from build123d import *

# Parameters (mm, degrees)
BOSS_EXTRUDE2_DEPTH      = 6.35
FILLET1_R                = 0.254
CIRPATTERN3_COUNT        = 3
FILLET1_OF_CIRPATTERN3_R = 0.254
CUT_EXTRUDE1_DEPTH       = 22.220069761
CUT_EXTRUDE1_DEPTH_BACK  = 22.220069761
SKETCH6_R                = 0.79375


with BuildPart() as part:
    # Sketch3 → Revolve1 (revolve)
    with BuildSketch(Plane.XY, mode=Mode.PRIVATE) as revolve1_sk:
        Polygon((0, 9.9568), (0, 2.4511), (15.875, 2.4511), (15.875, 4.0386), (3.175, 5.98805), (3.175, 9.9568), align=None)
    revolve(revolve1_sk.sketch.rotate(Axis((0, 0, 0), (1, 0, 0)), 90), axis=Axis((0, 0, 0), (1, 0, 0)))

    # Sketch5 → Boss-Extrude2 (add)
    with BuildSketch(Plane.ZY.offset(-15.875)):
        with BuildLine():
            ThreePointArc((-0.381, 2.421307541), (0, 2.4511), (0.381, 2.421307541))
            ThreePointArc((0.381, 2.421307541), (0, 2.3241), (-0.381, 2.421307541))
        make_face()
    boss_extrude2 = extrude(amount=BOSS_EXTRUDE2_DEPTH)

    # Fillet1
    # the kernel refuses this fillet: 0.254 mm, written as the material it takes off along each edge
    with BuildSketch(Plane(origin=(9.525, 3.119358803, 0), x_dir=(0, -0.2692049658318269, 0.9630829073197619), z_dir=(0, 0.9630829073197619, 0.2692049658318269))) as fillet1_piece_1_section:
        with BuildLine():
            CenterArc((0.795258803 - FILLET1_R, FILLET1_R), FILLET1_R, 270, 90)
            Line((0.795258803 - FILLET1_R, 0), (0.795258803, 0))
            Line((0.795258803, 0), (0.795258803, FILLET1_R))
        make_face()
    fillet1_piece_1 = revolve(axis=Axis((9.525, 3.119358803, 0), (1, 0, 0)), revolution_arc=148.766073655, mode=Mode.PRIVATE)
    fillet1_piece_1 = fillet1_piece_1 & Plane(origin=(9.597702858, 0, 0), x_dir=(0, 0, 1), z_dir=(1, 0, 0)) * Cylinder(2.4511, 4, mode=Mode.PRIVATE)
    add(fillet1_piece_1, mode=Mode.SUBTRACT)

    # CirPattern3: Boss-Extrude2 ×3 about axis
    cirpattern3_axis = Axis((0, 0, 0), (1, 0, 0))
    for i in range(1, CIRPATTERN3_COUNT):
        add(boss_extrude2.rotate(cirpattern3_axis, i * 360 / CIRPATTERN3_COUNT))

    # Fillet1 of CirPattern3
    # the kernel refuses this fillet: 0.254 mm, written as the material it takes off along each edge
    with BuildSketch(Plane(origin=(9.525, -1.559679402, 2.701443967), x_dir=(0, -0.699451780773575, -0.7146797928951643), z_dir=(0, -0.7146797928951643, 0.699451780773575))) as fillet1_of_cirpattern3_piece_1_section:
        with BuildLine():
            CenterArc((0.795258803 - FILLET1_OF_CIRPATTERN3_R, FILLET1_OF_CIRPATTERN3_R), FILLET1_OF_CIRPATTERN3_R, 270, 90)
            Line((0.795258803 - FILLET1_OF_CIRPATTERN3_R, 0), (0.795258803, 0))
            Line((0.795258803, 0), (0.795258803, FILLET1_OF_CIRPATTERN3_R))
        make_face()
    fillet1_of_cirpattern3_piece_1 = revolve(axis=Axis((9.525, -1.559679402, 2.701443967), (1, 0, 0)), revolution_arc=148.766073655, mode=Mode.PRIVATE)
    fillet1_of_cirpattern3_piece_1 = fillet1_of_cirpattern3_piece_1 & Plane(origin=(9.597702858, 0, 0), x_dir=(0, 0, 1), z_dir=(1, 0, 0)) * Cylinder(2.4511, 4, mode=Mode.PRIVATE)
    add(fillet1_of_cirpattern3_piece_1, mode=Mode.SUBTRACT)
    with BuildSketch(Plane(origin=(9.525, -1.559679402, -2.701443967), x_dir=(0, 0.968656746605401, -0.24840311442459811), z_dir=(0, -0.24840311442459811, -0.968656746605401))) as fillet1_of_cirpattern3_piece_2_section:
        with BuildLine():
            CenterArc((0.795258803 - FILLET1_OF_CIRPATTERN3_R, FILLET1_OF_CIRPATTERN3_R), FILLET1_OF_CIRPATTERN3_R, 270, 90)
            Line((0.795258803 - FILLET1_OF_CIRPATTERN3_R, 0), (0.795258803, 0))
            Line((0.795258803, 0), (0.795258803, FILLET1_OF_CIRPATTERN3_R))
        make_face()
    fillet1_of_cirpattern3_piece_2 = revolve(axis=Axis((9.525, -1.559679402, -2.701443967), (1, 0, 0)), revolution_arc=148.766073655, mode=Mode.PRIVATE)
    fillet1_of_cirpattern3_piece_2 = fillet1_of_cirpattern3_piece_2 & Plane(origin=(9.597702858, 0, 0), x_dir=(0, 0, 1), z_dir=(1, 0, 0)) * Cylinder(2.4511, 4, mode=Mode.PRIVATE)
    add(fillet1_of_cirpattern3_piece_2, mode=Mode.SUBTRACT)

    # Sketch6 → Cut-Extrude1 (cut, two sides: drawn at the far end of the back side and taken through both)
    with BuildSketch(Plane.XY.offset(-CUT_EXTRUDE1_DEPTH_BACK)):
        with Locations((7.9375, 0)):
            Circle(SKETCH6_R)
    extrude(amount=CUT_EXTRUDE1_DEPTH + CUT_EXTRUDE1_DEPTH_BACK, mode=Mode.SUBTRACT)


solid = part.part
Can you work these out from the model? Positions are in its coordinate system, mm. A direction names the side the tool comes from. Coordinates: 2 decimals unless noted, no trailing zeros. Write each loop counter-clockwise with the first axis right and the second up, starting at its lowest first coordinate (ties: lowest second). Pieces come first, ordered by that corner, then holes. Notation, with made-up numbers: (17.5, 83) -> (56.5, 83) arc R27 cw to (56.5, 102) -> close; hole circle Ø5 at (48, -17.5). An arc over 180 degrees is marked (long way). Write each question's results on one line, items separated by ' | '. Start each with the question number.
Q1. We'd pull the mould along X, two halves only. Please class faces 1 (the face through (7.145, 0.035, 3.827)), 2 (the face through (7.145, 0.035, -3.87)), 3 (the face through (0, 2, 2)), 4 (the face through (10.85, -1.44, 4.59)): +X half, -X half, draft (parallel to the pull), parting line (faces both ways), or undercut.
Q2. On a 3-axis mill with a long thin cutter (end or side, diameter ignored), from which of +Z, -Z, +X, -X, +Y, -Y can I reach the whole of each face in a straight line? I mean faces 5 (the face through (3.175, -0.1, -6.5)), 6 (the face through (1.565, -2.991, 9.497)). Say none if no direction works.
Q3. I'm going to push flat-ended pins straight in: pin 1 (4 mm diameter, centred on y = 6, z = -5, fed in from -X); pin 2 (2.5 mm diameter, centred on x = 7.94, y = 0, fed in from -Z); pin 3 (5 mm diameter, centred on x = 4.5, y = -7, fed in from +Z); pin 4 (2.5 mm diameter, centred on x = 7.94, y = 0, fed in from +Z). Where does each tip first touch, or does it pass through?
Q4. Imagine slicing it at B-B (y = 0). Write out the boundary of the cut face in (x, z) (3 decimals).
Q5. Imagine slicing it at D-D (y = -7.5). Write out the boundary of the cut face in (x, z) (3 decimals).
Q6. Imagine slicing it at A-A (z = 0). Write out the boundary of the cut face in (x, y) (3 decimals).
Q7. Imagine slicing it at C-C (x = 5.5). Write out the boundary of the cut face in (y, z), then the cut area to 3 significant figures.
Q8. If I drill on probe 1 along X at (y, z) = (0, -3) (3 decimals); probe 2 along X at (y, z) = (3.5, 7) (3 decimals); probe 3 along Y at (x, z) = (9, 0), over which ranges is the centre line in solid material (lowest first)?
Taken from the geometry:
1) face 1: undercut | face 2: undercut | face 3: -X half | face 4: +X half
2) face 5: +X | face 6: +X, -X
3) pin 1: stops at x = 0 | pin 2: stops at z = -5.45 | pin 3: stops at z = 8.68 | pin 4: stops at z = 5.45
4) outline: (0, -9.957) -> (3.175, -9.957) -> (3.175, -5.988) -> (7.144, -5.379) -> (7.144, -2.451) -> (0, -2.451) -> close; (0, 2.451) -> (7.144, 2.451) -> (7.144, 5.379) -> (3.175, 5.988) -> (3.175, 9.957) -> (0, 9.957) -> close; (8.731, -5.135) -> (15.875, -4.039) -> (15.875, -2.451) -> (8.731, -2.451) -> close; (8.731, 2.451) -> (15.875, 2.451) -> (15.875, 4.039) -> (8.731, 5.135) -> close
5) outline: (0, -6.549) -> (3.175, -6.549) -> (3.175, 6.549) -> (0, 6.549) -> close
6) outline: (0, -9.957) -> (3.175, -9.957) -> (3.175, -5.988) -> (15.875, -4.039) -> (15.875, -2.451) -> (0, -2.451) -> close; (0, 2.451) -> (9.559, 2.451) arc R0.254 ccw to (9.779, 2.324) -> (15.875, 2.324) -> (15.875, 4.039) -> (3.175, 5.988) -> (3.175, 9.957) -> (0, 9.957) -> close
7) outline: circle Ø11.26 at (0, 0); hole circle Ø4.9 at (0, 0) | area: 80.7 mm^2
8) probe 1: x = 0 to 7.144, 8.731 to 15.875 | probe 2: x = 0 to 3.175 | probe 3: y = -5.09 to -2.45, 2.45 to 5.09
